The model under review builds one solid part; all positions refer to its coordinate system, in mm. A direction names the side the tool comes from. Coordinates: 2 decimals unless noted, no trailing zeros. Order: outer loops, then holes, each group sorted by start corner. A loop starts at its lowest first (then second) coordinate and runs counter-clockwise, first axis right, second up. Notation, with made-up numbers: (69.25, -24) -> (104.25, -24) arc R30 ccw to (104.25, -2) -> close; hole circle Ø5 at (38, 40.25). An arc over 180 degrees is marked (long way). Use one line per item in the form item = value.
Autodesk Inventor part; units mm, degrees
ref_plane "工作平面1" through (0, 10, 0) normal (0, 1, 0) x (-1, 0, 0)
ref_plane "工作平面2" through (0, -7.5, 450) normal (0, 1, 0) x (-1, 0, 0)
ref_plane "YZ Plane" through (0, 0, 0) normal (1, 0, 0) x (0, 1, 0)
sketch "草图1" plane through (0, 0, 0) normal (0, 0, 1) x (1, 0, 0)
  circle A0 centre (0, 0) radius 10
  dimension "d0" = 20
extrude "拉伸1" add sketch "草图1" along normal blind 450
sketch "草图2" plane through (0, 0, 450) normal (0, 0, 1) x (1, 0, 0)
  circle A0 centre (0, 0) radius 7.5
  dimension "d3" = 15
extrude "拉伸2" add sketch "草图2" along normal blind 40
sketch "草图3" plane through (0, 0, 0) normal (0, 0, -1) x (-1, 0, 0)
  circle A0 centre (0, 0) radius 7.5
  dimension "d6" = 15
extrude "拉伸3" add sketch "草图3" along normal blind 15
chamfer "倒角1" distance 0.5 angle 45 1 edges at (7.5, 0, -15)
ref_plane "工作平面1" through (0, 10, 0) normal (0, 1, 0) x (-1, 0, 0)
sketch "草图4" plane through (0, 10, 0) normal (0, 1, 0) x (-1, 0, 0)
  line L0 (3, 392) -> (-3, 392)
  line L1 (-3, 392) -> (-3, 408)
  line L2 (-3, 408) -> (3, 408)
  line L3 (3, 408) -> (3, 392)
  arc A0 (-3, 392) -> (3, 392) centre (0, 392) ccw
  arc A1 (3, 408) -> (-3, 408) centre (0, 408) ccw
  line L4 (10, 450) -> (-10, 450)
  point P0 (0, 0)
  dimension "d12" = 6
  dimension "d13" = 16
  dimension "d14" = 0
  dimension "d15" = 42
extrude "拉伸4" cut sketch "草图4" against normal blind 2.5
pattern_linear "矩形阵列1" count 4 spacing 120 along (0, 0, -1) of "拉伸4"
ref_plane "工作平面2" through (0, -7.5, 450) normal (0, 1, 0) x (-1, 0, 0)
sketch "草图5" plane through (0, -7.5, 450) normal (0, 1, 0) x (-1, 0, 0)
  circle A0 centre (0, 30) radius 2
  line L0 (7.5, 40) -> (-7.5, 40)
  line L1 (0, -450) -> (0, -436.617)
  dimension "d21" = 4
  dimension "d22" = 10
  dimension "d23" = 13.383
extrude "拉伸5" cut sketch "草图5" along normal blind 1.5
properties part number "砂轮轴"
Item 1: We need section A-A (y = 0). Write out the cut boundary in (x, z), plus the area to 3 significant figures.
Results found:
outline = (-10, 0) -> (-7.5, 0) -> (-7.5, -14.5) -> (-7, -15) -> (7, -15) -> (7.5, -14.5) -> (7.5, 0) -> (10, 0) -> (10, 450) -> (7.5, 450) -> (7.5, 490) -> (-7.5, 490) -> (-7.5, 450) -> (-10, 450) -> close
area = 9,820 mm²
Item 2: We need section B-B (z = 264.5). Write out the cut boundary in (x, y), plus the area to 3 significant figures.
Results found:
outline = circle Ø20 at (0, 0)
area = 314 mm²
Item 3: Tool access review of faces 1 (the face through (0, 0, 490)), 2 (the face through (4, 7, 0)), 3 (the face through (4, 7, 450)): name each direction out of +Z, -Z, +X, -X, +Y, -Y from which nothing blocks a thin tool from reaching the whole face with its end or side.
Results found:
face_1 = +Z, +X, -X, +Y, -Y
face_2 = -Z
face_3 = +Z
Item 4: Clearance check with flat-ended pins moving along their axes: pin 1 (5 mm diameter, centred on x = -1, z = 397, fed in from +Y); pin 2 (1.6 mm diameter, centred on y = 8.5, z = 39, fed in from +X); pin 3 (2 mm diameter, centred on y = 9, z = 284, fed in from -X). State where each tip first meets the part, or that it passes through.
Results found:
pin_1 = 9.54
pin_2 = 6.38
pin_3 = -6
Item 5: To check wall thickness, follow L1, parallel to Z at x = 0, y = -6.5; L2, parallel to Z at x = -2.25, y = 8; L3, parallel to Z at x = 0, y = -7.05. State the ranges of each line that lie inside material, in increasing order. Write a range as from..to.
Results found:
L1 = -15..478, 482..490
L2 = 0..30.02, 49.98..150.02, 169.98..270.02, 289.98..390.02, 409.98..450
L3 = -14.95..478, 482..490
